The listing builds one solid part. Answer for the finished solid, in the listing's coordinates (mm). A direction names the side the tool comes from. Coordinates: 2 decimals unless noted, no trailing zeros. Loops run counter-clockwise (first coordinate to the right, second up) from the corner with the lowest first, then second, coordinate; pieces in that order, holes last. Notation, with made-up numbers: (10, 33) - (40, 33) arc R20 ccw to (40, 51) - close; hole circle Ø9 at (-12.75, 13.5). An arc over 180 degrees is marked (long way). Return JSON: item names as keys, results as strings. Group by question number.
1. Section B-B (y = 63.5) is taken. Write down the section's boundary in (x, z).
2. Find the intervals of material crossed by line 1 along Z through (x, y) = (286, 63.5); line 2 along Y through (x, z) = (188.5, 24.5); line 3 along Y through (x, z) = (236.5, 32), in increasing order.
3. Section C-C (z = 70.5) is taken. Write down the section's boundary in (x, y).
4. Which of the six approach directions +Z, -Z, +X, -X, +Y, -Y give full straight-line access (tool end or side, diameter ignored) to faces 1 (the face through (286, 64, 38.1)), 2 (the face through (286.017, 28.983, 70.171)), 3 (the face through (170, 41, 16.51)), 4 (the face through (266.7, 63, 63))?
5. The mould has two halves that part along Y. Classify faces 5 (the face through (150, 77, 0)), 6 (the face through (170, 86, 29.21)), 7 (the face through (170, 31.75, 23)), 8 (the face through (116, 0, 29)): pulls with the +Y half, pulls with the -Y half, needs draft (parallel to the pull), parting line crosses it, or undercut.
6. Section A-A (x = 146) is taken. Write down the section's boundary in (y, z).
7. Each of these flat-tipped pins is pushed along its axis until it touches: P1, Ø3, axis at x = 111, y = 29, coming from the +Z side; P2, Ø17.5, axis at x = 285.5, y = 10.5, coming from the +Z side; P3, Ø5, axis at x = 281, y = 121.5, coming from the +Z side; P4, Ø12, axis at x = 244, y = 70, coming from the -Z side. Where does it stop, or does it pass through?
8. Section D-D (y = 11) is taken. Write down the section's boundary in (x, z).
```python
from build123d import *

# Parameters (mm, degrees)
F0_W     = 38.1
F0_H     = 50.8
F1_DEPTH = 127
F2_SIZE2 = 19.05
F2_SIZE  = 19.05
F4_DEPTH = 273.05
F3_R     = 12.7
F5_DEPTH = 38.1
F6_DEPTH = 38.1


with BuildPart() as f1:
    # F0 (on Front) → F1 (new body)
    with BuildSketch(Plane.XZ):
        Polygon((0, 101.6), (0, 0), (304.8, 0), (304.8, 50.8), (266.7, 50.8), (266.7, 38.1), (31.75, 38.1), (31.75, 101.6), align=None)
        with Locations((285.75, 76.2)):
            Rectangle(F0_W, F0_H)
    extrude(amount=-F1_DEPTH)

    # F2
    f2_edges = [f1.edges().sort_by_distance(p)[0] for p in [
        (0, 63.5, 101.6),
    ]]
    chamfer(f2_edges, length=F2_SIZE, length2=F2_SIZE2)

    # F3 (on face) → F4 (cut, through all)
    with BuildSketch(Plane.YZ.offset(304.8)):
        Polygon((50.8, 16.51), (50.8, 0), (63.5, 0), (76.2, 0), (76.2, 16.51), (95.25, 16.51), (95.25, 29.21), (76.2, 29.21), (76.2, 38.1), (63.5, 38.1), (50.8, 38.1), (50.8, 29.21), (31.75, 29.21), (31.75, 16.51), align=None)
    extrude(amount=-F4_DEPTH, mode=Mode.SUBTRACT)

    # F3 (on face) → F5 (cut)
    with BuildSketch(Plane.YZ.offset(304.8)):
        with Locations((63.5, 76.2)):
            Circle(F3_R)
    extrude(amount=-F5_DEPTH, mode=Mode.SUBTRACT)

    # F3 (on face) → F6 (cut)
    with BuildSketch(Plane.YZ.offset(304.8)):
        with BuildLine():
            Line((0, 101.6), (0, 50.8))
            Line((0, 50.8), (15.875, 50.8))
            Line((15.875, 50.8), (42.463992, 90.091243))
            ThreePointArc((42.463992, 90.091243), (63.5, 101.255851), (84.536008, 90.091243))
            Line((84.536008, 90.091243), (111.125, 50.8))
            Line((111.125, 50.8), (127, 50.8))
            Line((127, 50.8), (127, 101.6))
            Line((127, 101.6), (0, 101.6))
        make_face()
    extrude(amount=-F6_DEPTH, mode=Mode.SUBTRACT)


solid = f1.part
```
The answers:
{
 "1": {"outline": "(0, 0) - (31.75, 0) - (31.75, 101.6) - (19.05, 101.6) - (0, 82.55) - close; (266.7, 38.1) - (304.8, 38.1) - (304.8, 63.5) - (266.7, 63.5) - close; (266.7, 88.9) - (304.8, 88.9) - (304.8, 101.26) - (266.7, 101.26) - close"},
 "2": {"line 1": "z = 38.1 to 63.5, 88.9 to 101.26", "line 2": "y = 0 to 31.75, 95.25 to 127", "line 3": "y = 0 to 50.8, 76.2 to 127"},
 "3": {"outline": "(0, 0) - (31.75, 0) - (31.75, 127) - (0, 127) - close; (266.7, 29.21) - (304.8, 29.21) - (304.8, 52.15) - (266.7, 52.15) - close; (266.7, 74.85) - (304.8, 74.85) - (304.8, 97.79) - (266.7, 97.79) - close"},
 "4": {"face 1": "-Z, +X", "face 2": "+Z, +X, -Y", "face 3": "+X", "face 4": "+Z, +Y, -Y"},
 "5": {"face 5": "needs draft", "face 6": "undercut", "face 7": "undercut", "face 8": "pulls with the -Y half"},
 "6": {"outline": "(0, 0) - (50.8, 0) - (50.8, 16.51) - (31.75, 16.51) - (31.75, 29.21) - (50.8, 29.21) - (50.8, 38.1) - (0, 38.1) - close; (76.2, 0) - (127, 0) - (127, 38.1) - (76.2, 38.1) - (76.2, 29.21) - (95.25, 29.21) - (95.25, 16.51) - (76.2, 16.51) - close"},
 "7": {"P1": "stops at z = 38.1", "P2": "stops at z = 55.79", "P3": "stops at z = 50.8", "P4": "passes through"},
 "8": {"outline": "(0, 0) - (304.8, 0) - (304.8, 50.8) - (266.7, 50.8) - (266.7, 38.1) - (31.75, 38.1) - (31.75, 101.6) - (19.05, 101.6) - (0, 82.55) - close"}
}
